Design review of the part built by this model. Coordinates are the model's own, in mm. Face numbers are marked on the shaded views. A direction names the side the tool comes from. Round coordinates to 2 decimals unless told otherwise and drop trailing zeros. Write each loop counter-clockwise with the first axis right and the second up, starting at its lowest first coordinate (ties: lowest second). Pieces come first, ordered by that corner, then holes.
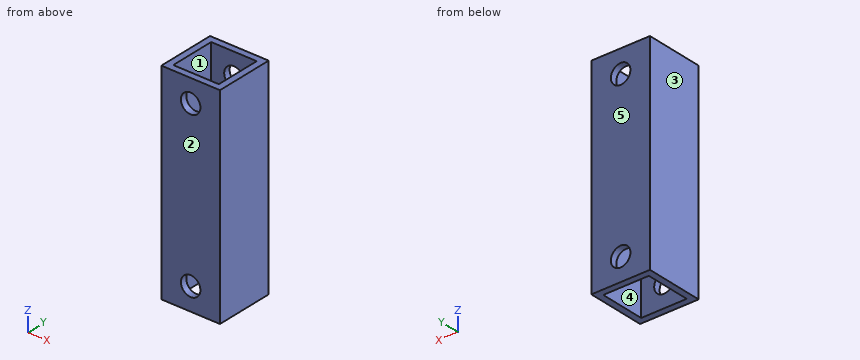
from build123d import *

# Parameters (mm, degrees)
SKETCH_1_W          = 9
SKETCH_1_H          = 9
EXTRUDE_1_DEPTH     = 32
SKETCH_2_W          = 7
SKETCH_2_H          = 7
CUT_EXTRUDE_1_DEPTH = 40
SKETCH_3_R          = 1.5
CUT_EXTRUDE_2_DEPTH = 38


with BuildPart() as part:
    # ｽｹｯﾁ1 → ﾎﾞｽ - 押し出し1 (new body)
    with BuildSketch(Plane.XY):
        Rectangle(SKETCH_1_W, SKETCH_1_H)
    extrude(amount=EXTRUDE_1_DEPTH)

    # ｽｹｯﾁ2 → ｶｯﾄ - 押し出し1 (cut)
    with BuildSketch(Plane.XY.offset(32)):
        Rectangle(SKETCH_2_W, SKETCH_2_H)
    extrude(amount=-CUT_EXTRUDE_1_DEPTH, mode=Mode.SUBTRACT)

    # ｽｹｯﾁ3 → ｶｯﾄ - 押し出し2 (cut)
    with BuildSketch(Plane(origin=(0, 4.5, 0), x_dir=(1, 0, 0), z_dir=(0, 1, 0))):
        with Locations((0, -3.5)):
            Circle(SKETCH_3_R)
        with Locations((0, -28.5)):
            Circle(SKETCH_3_R)
    extrude(amount=-CUT_EXTRUDE_2_DEPTH, mode=Mode.SUBTRACT)


solid = part.part
1) Add section B-B on z = 3.5. State the section outline as (x, y) points.
2) Add section A-A on x = 0. State the section outline as (y, z) points.
3) For P1, Ø1.8, axis at x = 0, z = 3.5, coming from the -Y side, flat-tipped, find the tip position at first contact; note if it passes through.
4) Add section C-C on y = -2.25. State the section outline as (x, z) points, and give its area (3 significant figures).
5) For line 1 along Z through (x, y) = (0, 3.9); line 2 along X through (y, z) = (-2.5, 28), list the stretches that pass through material, from the lowest coordinate up.
6) The part is to be moulded in two halves that separate along X. For the marked faces 1, 2 and 3, say which applies: pulls with the +X half, pulls with the -X half, needs draft (parallel to the pull), parting line crosses it, or undercut.
7) For the marked faces 4 and 5, list the 3-axis set-ups (+Z, -Z, +X, -X, +Y, -Y) from which the entire face can be reached by the end or side of a thin tool; tool diameter is ignored.
Computed:
1. outline: (-4.5, -4.5) - (-1.5, -4.5) - (-1.5, -3.5) - (-3.5, -3.5) - (-3.5, 3.5) - (-1.5, 3.5) - (-1.5, 4.5) - (-4.5, 4.5) - close; (1.5, -4.5) - (4.5, -4.5) - (4.5, 4.5) - (1.5, 4.5) - (1.5, 3.5) - (3.5, 3.5) - (3.5, -3.5) - (1.5, -3.5) - close
2. outline: (-4.5, 0) - (-3.5, 0) - (-3.5, 2) - (-4.5, 2) - close; (-4.5, 5) - (-3.5, 5) - (-3.5, 27) - (-4.5, 27) - close; (-4.5, 30) - (-3.5, 30) - (-3.5, 32) - (-4.5, 32) - close; (3.5, 0) - (4.5, 0) - (4.5, 2) - (3.5, 2) - close; (3.5, 5) - (4.5, 5) - (4.5, 27) - (3.5, 27) - close; (3.5, 30) - (4.5, 30) - (4.5, 32) - (3.5, 32) - close
3. P1: passes through
4. outline: (-4.5, 0) - (-3.5, 0) - (-3.5, 32) - (-4.5, 32) - close; (3.5, 0) - (4.5, 0) - (4.5, 32) - (3.5, 32) - close
4. area: 64.0 mm2
5. line 1: z = 0 to 2, 5 to 27, 30 to 32
5. line 2: x = -4.5 to -3.5, 3.5 to 4.5
6. face 1: undercut
6. face 2: needs draft
6. face 3: pulls with the -X half
7. face 4: +Z, -Z
7. face 5: +Z, -Z, +X, -X, +Y
